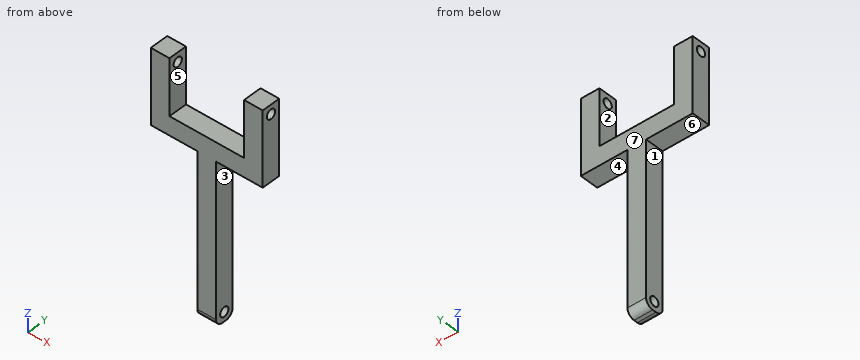
```python
from build123d import *

# Parameters (mm, degrees)
SKETCH1_W                = 12.7
SKETCH1_H                = 12.7
BOSS_EXTRUDE1_DEPTH      = 41.656
BOSS_EXTRUDE1_DEPTH_BACK = 80.01
SKETCH4_W                = 12.7
SKETCH4_H                = 12.7
BOSS_EXTRUDE2_DEPTH      = 38.1
SKETCH5_W                = 12.7
SKETCH5_H                = 12.7
BOSS_EXTRUDE3_DEPTH      = 50.8
SKETCH6_R                = 3.175
CUT_EXTRUDE1_DEPTH       = 16.51
SKETCH7_R                = 3.175
CUT_EXTRUDE2_DEPTH       = 45.45
FILLET1_R                = 5.08


with BuildPart() as part:
    # Sketch1 → Boss-Extrude1 (new body, two sides)
    with BuildSketch(Plane.XY) as boss_extrude1_sk:
        Rectangle(SKETCH1_W, SKETCH1_H)
    extrude(amount=BOSS_EXTRUDE1_DEPTH)
    extrude(boss_extrude1_sk.sketch, amount=-BOSS_EXTRUDE1_DEPTH_BACK)

    # Sketch4 → Boss-Extrude2 (add, symmetric)
    with BuildSketch(Plane(origin=(0, 0, 0), x_dir=(0, 0, -1), z_dir=(1, 0, 0))):
        with Locations((-35.306, 0)):
            Rectangle(SKETCH4_W, SKETCH4_H)
    extrude(amount=BOSS_EXTRUDE2_DEPTH, both=True)

    # Sketch5 → Boss-Extrude3 (add)
    with BuildSketch(Plane(origin=(0, 0, 28.956), x_dir=(-1, 0, 0), z_dir=(0, 0, -1))):
        with Locations((-31.75, 0)):
            Rectangle(SKETCH5_W, SKETCH5_H)
    boss_extrude3 = extrude(amount=-BOSS_EXTRUDE3_DEPTH)

    # Sketch6 → Cut-Extrude1 (cut)
    with BuildSketch(Plane.ZY.offset(-25.4)):
        with Locations((73.406, 0)):
            Circle(SKETCH6_R)
    cut_extrude1 = extrude(amount=-CUT_EXTRUDE1_DEPTH, mode=Mode.SUBTRACT)

    # Mirror1: Boss-Extrude3, Cut-Extrude1 across plane
    add(boss_extrude3.mirror(Plane(origin=(0, 0, 0), x_dir=(0, 0, 1), z_dir=(1, 0, 0))))
    add(cut_extrude1.mirror(Plane(origin=(0, 0, 0), x_dir=(0, 0, 1), z_dir=(1, 0, 0))), mode=Mode.SUBTRACT)

    # Sketch7 → Cut-Extrude2 (cut, through all)
    with BuildSketch(Plane.ZY.offset(6.35)):
        with Locations((-73.66, 0)):
            Circle(SKETCH7_R)
    extrude(amount=-CUT_EXTRUDE2_DEPTH, mode=Mode.SUBTRACT)

    # Fillet1
    fillet1_edges = [part.edges().sort_by_distance(p)[0] for p in [
        (0, 6.35, -80.01),
        (0, -6.35, -80.01),
    ]]
    fillet(fillet1_edges, radius=FILLET1_R)


solid = part.part
```
Check sheet for the modelled part. Datum: model origin and axes. Units: mm. Face numbers are marked on the shaded views. A direction names the side the tool comes from. Round coordinates to 2 decimals unless told otherwise and drop trailing zeros. Loops run counter-clockwise (first coordinate to the right, second up) from the corner with the lowest first, then second, coordinate; pieces in that order, holes last. Notation, with made-up numbers: (19.25, 51) - (44.25, 51) arc R6 ccw to (44.25, 56) - close; hole circle Ø11 at (76, 75.25). An arc over 180 degrees is marked (long way). Write item = value, one per line. Start each with the question number.
Q1. Release check for a two-part mould opening along X. For the marked faces 1, 2 and 3 record: pulls with the +X half, pulls with the -X half, needs draft (parallel to the pull), parting line crosses it, or undercut.
Q2. Thickness scan on L1, parallel to X at y = 2.5, z = 49; L2, parallel to X at y = 2.5, z = -59.5; L3, parallel to Z at x = 11, y = 3.75. Record the ranges inside material, lowest first.
Q3. Section check B-B (x = -20.5). Record the boundary of the cut face in (y, z), plus the area to 3 significant figures.
Q4. Section check A-A (z = 60.5). Record the boundary of the cut face in (x, y), plus the area to 3 significant figures.
Q5. Access from +Z, -Z, +X, -X, +Y, -Y to the whole of each face (thin tool, end or side, straight path). Record for the marked faces 4, 5, 6 and 7.
Q6. Section check C-C (z = -9.5). Record the boundary of the cut face in (x, y).
Q7. Depth check by flat-ended pin: P1, Ø4, axis at x = -13.5, y = -3.5, coming from the -Z side; P2, Ø2, axis at x = -23, y = -1.5, coming from the +Z side; P3, Ø4, axis at y = -1, z = -41.5, coming from the +X side. Enter the tip coordinate at first touch or a pass-through.
Derived:
q1.face_1 = pulls with the -X half
q1.face_2 = undercut
q1.face_3 = pulls with the +X half
q2.L1 = -38.1 to -25.4, 25.4 to 38.1
q2.L2 = -6.35 to 6.35
q2.L3 = 28.96 to 41.66
q3.outline = (-6.35, 28.96) - (6.35, 28.96) - (6.35, 41.66) - (-6.35, 41.66) - close
q3.area = 161 mm^2
q4.outline = (-38.1, -6.35) - (-25.4, -6.35) - (-25.4, 6.35) - (-38.1, 6.35) - close; (25.4, -6.35) - (38.1, -6.35) - (38.1, 6.35) - (25.4, 6.35) - close
q4.area = 323 mm^2
q5.face_4 = -Z, +X, +Y, -Y
q5.face_5 = +Z, +Y, -Y
q5.face_6 = -Z, -X, +Y, -Y
q5.face_7 = +Z, -Z, +X, -X, +Y
q6.outline = (-6.35, -6.35) - (6.35, -6.35) - (6.35, 6.35) - (-6.35, 6.35) - close
q7.P1 = 28.96
q7.P2 = 41.66
q7.P3 = 6.35
